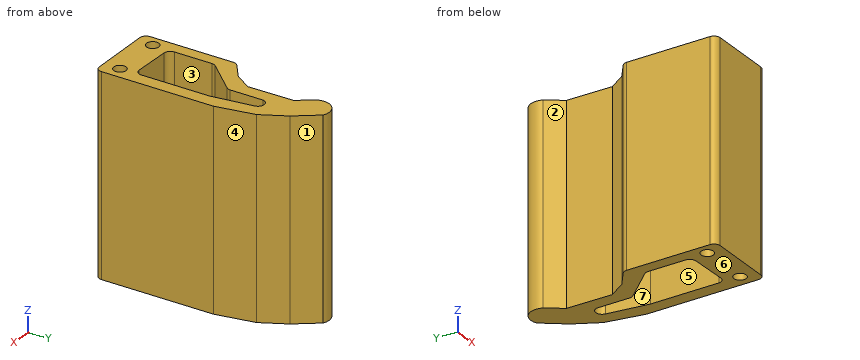
from build123d import *

# Parameters (mm, degrees)
BOSS_EXTRUDE1_DEPTH = 32
FILLET1_R           = 1
SKETCH2_R           = 1
CUT_EXTRUDE1_DEPTH  = 32


with BuildPart() as part:
    # Sketch1 → Boss-Extrude1 (new body)
    with BuildSketch(Plane.XY.offset(40)):
        with BuildLine():
            Line((-312.030492528, 377.868524993), (-310.193868717, 375.244776692))
            Line((-310.193868717, 375.244776692), (-310.096008301, 367.875213623))
            Line((-310.096008301, 367.875213623), (-311.889068604, 365.166412354))
            Line((-311.889068604, 365.166412354), (-314.88168335, 362.936676025))
            Line((-314.88168335, 362.936676025), (-314.88168335, 347.918438133))
            Line((-314.88168335, 347.918438133), (-302.847373473, 347.918438133))
            Line((-302.847373473, 347.918438133), (-302.847373473, 367.04556325))
            Line((-302.847373473, 367.04556325), (-304.028060208, 373.263846724))
            Line((-304.028060208, 373.263846724), (-306.153296332, 377.278181625))
            Line((-306.153296332, 377.278181625), (-308.864528411, 380.917030307))
            ThreePointArc((-308.864528411, 380.917030307), (-311.535911341, 380.523114569), (-312.030492528, 377.868524993))
        make_face()
        with BuildLine():
            Line((-312.988408734, 360.598376943), (-312.988408734, 353.109979303))
            Line((-312.988408734, 353.109979303), (-305, 352.927314193))
            Line((-305, 352.927314193), (-305, 365))
            Line((-305, 365), (-305.952850342, 371.670013428))
            ThreePointArc((-305.952850342, 371.670013428), (-306.959348498, 372.584855641), (-307.99460106, 371.702683918))
            Line((-307.99460106, 371.702683918), (-307.99460106, 366.023339102))
            Line((-307.99460106, 366.023339102), (-312.988408734, 360.598376943))
        make_face(mode=Mode.SUBTRACT)
    extrude(amount=BOSS_EXTRUDE1_DEPTH)

    # Fillet1
    fillet1_edges = [part.edges().sort_by_distance(p)[0] for p in [
        (-302.847373473, 347.918438133, 56),
        (-314.88168335, 347.918438133, 56),
        (-314.88168335, 362.936676025, 56),
        (-307.99460106, 366.023339102, 56),
        (-312.988408734, 360.598376943, 56),
        (-312.988408734, 353.109979303, 56),
        (-305, 352.927314193, 56),
    ]]
    fillet(fillet1_edges, radius=FILLET1_R)

    # Sketch2 → Cut-Extrude1 (cut)
    with BuildSketch(Plane.XY.offset(72)):
        with Locations((-313.031111026, 350.560286037)):
            Circle(SKETCH2_R)
        with Locations((-304.91451991, 350.560286037)):
            Circle(SKETCH2_R)
    extrude(amount=-CUT_EXTRUDE1_DEPTH, mode=Mode.SUBTRACT)


solid = part.part
Part model, mm, in its own coordinate system. Face numbers are marked on the shaded views. A direction names the side the tool comes from. Coordinates: 2 decimals unless noted, no trailing zeros. Write each loop counter-clockwise with the first axis right and the second up, starting at its lowest first coordinate (ties: lowest second). Pieces come first, ordered by that corner, then holes. Notation, with made-up numbers: M -37.5,36.5 L -6.5,36.5 A29 ccw -6.5,61.5 Z; hole C -28.75,33.25 d2. An arc over 180 degrees is marked long. Return JSON: item names as keys, results as strings.
1. Pull direction X, two halves, no side cores. Call the marked faces 4, 5, 6 and 7: pulls with the +X half, pulls with the -X half, needs draft (parallel to the pull), parting line crosses it, or undercut.
Determined:
{"face 4": "pulls with the +X half", "face 5": "undercut", "face 6": "needs draft", "face 7": "undercut"}
2. 3-axis set-ups, long thin cutter, end or side, ignore diameter. For the marked faces 1, 2 and 3: which of +Z, -Z, +X, -X, +Y, -Y reach the whole face in a straight line?
Determined:
{"face 1": "+Z, -Z, +X, +Y", "face 2": "+Z, -Z, -X", "face 3": "+Z, -Z"}
3. Saw through at C-C, the plane z = 55. Write the cut outline in (x, y).
Determined:
{"outline": "M -314.88,348.92 A1 ccw -313.88,347.92 L -303.85,347.92 A1 ccw -302.85,348.92 L -302.85,367.05 L -304.03,373.26 L -306.15,377.28 L -308.86,380.92 A2.32 ccw -312.03,377.87 L -310.19,375.24 L -310.1,367.88 L -311.89,365.17 L -314.48,363.24 A1 ccw -314.88,362.43 Z; hole C -313.03,350.56 d2; hole M -312.99,354.09 A1 ccw -312.01,353.09 L -306.02,352.95 A1 ccw -305,353.95 L -305,365 L -305.95,371.67 A1.03 ccw -307.99,371.7 L -307.99,366.41 A1 cw -308.26,365.74 L -312.72,360.89 A1 ccw -312.99,360.21 Z; hole C -304.91,350.56 d2"}
4. Saw through at B-B, the plane x = -309.25. Write the cut outline in (y, z), then the cut area to 3 significant figures.
Determined:
{"outline": "M 347.92,40 L 353.02,40 L 353.02,72 L 347.92,72 Z; M 364.66,40 L 381.07,40 L 381.07,72 L 364.66,72 Z", "area": "689 mm²"}
5. Saw through at A-A, the plane y = 359.5. Write the cut outline in (x, z), then the cut area to 3 significant figures.
Determined:
{"outline": "M -314.88,40 L -312.99,40 L -312.99,72 L -314.88,72 Z; M -305,40 L -302.85,40 L -302.85,72 L -305,72 Z", "area": "129 mm²"}
6. Probe L1, parallel to Y at x = -312.75, z = 70; L2, parallel to X at y = 355.5, z = 60.5; L3, parallel to Y at x = -312, z = 68. List the from-to ranges inside material, lowest first.
Determined:
{"L1": "347.92 to 349.6, 351.52 to 353.44, 360.86 to 364.52", "L2": "-314.88 to -312.99, -305 to -302.85", "L3": "347.92 to 353.09, 361.67 to 365.08, 377.82 to 379.89"}
7. Saw through at D-D, the plane y = 378.5. Write the cut outline in (x, z).
Determined:
{"outline": "M -312.22,40 L -307.06,40 L -307.06,72 L -312.22,72 Z"}
8. Flat gauge pins, fed straight in: pin 1 Ø1.2 at (x, y) = (-304.91, 350.56) entering from -Z; pin 2 Ø1.5 at (y, z) = (373.5, 56) entering from -X; pin 3 Ø1.5 at (x, z) = (-307, 49.5) entering from +Y; pin 4 Ø3 at (x, z) = (-305.5, 44) entering from +Y. Where does each tip first touch, or does it go through?
Determined:
{"pin 1": "through", "pin 2": "x = -310.18", "pin 3": "y = 379.42", "pin 4": "y = 378.41"}
